Work out the finished part from the listing and answer in its coordinate system (mm). Round coordinates to 2 decimals unless told otherwise and drop trailing zeros. Loops run counter-clockwise (first coordinate to the right, second up) from the corner with the lowest first, then second, coordinate; pieces in that order, holes last. Notation, with made-up numbers: (-35, 45.25) - (-3, 45.25) arc R15 ccw to (-3, 59.25) - close; hole circle Ø3 at (5, 34). An arc over 180 degrees is marked (long way). Answer as CSV lines item,"result". Start each with the question number.
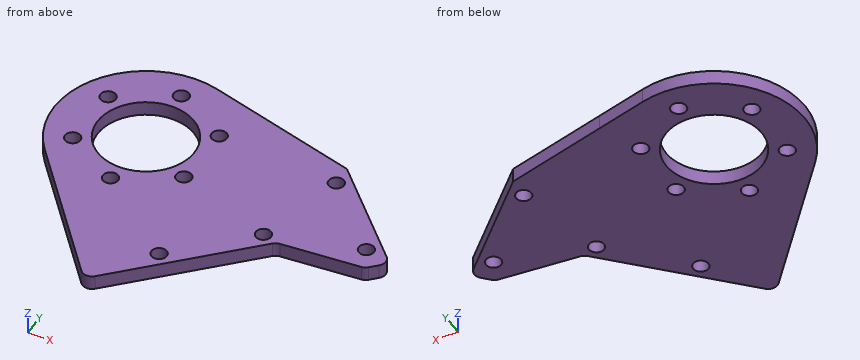
```python
from build123d import *

# Parameters (mm, degrees)
SKETCH_1_R          = 19
SKETCH_1_R_2        = 1.6
SKETCH_1_R_3        = 10
EXTRUDE_1_DEPTH     = 3
EXTRUDE_START       = -3
SKETCH_2_R          = 1.6
EXTRUDE_2_DEPTH     = 3
CUT_EXTRUDE_START   = -10
CUT_EXTRUDE_1_DEPTH = 10
EXTRUDE_4_DEPTH     = 3


with BuildPart() as part:
    # 草图1 → 凸台-拉伸1 (new body)
    with BuildSketch(Plane.XY):
        Circle(SKETCH_1_R)
        with Locations((0, 13.5)):
            Circle(SKETCH_1_R_2, mode=Mode.SUBTRACT)
        Circle(SKETCH_1_R_3, mode=Mode.SUBTRACT)
        with Locations((11.691342951, 6.75)):
            Circle(SKETCH_1_R_2, mode=Mode.SUBTRACT)
        with Locations((11.691342951, -6.75)):
            Circle(SKETCH_1_R_2, mode=Mode.SUBTRACT)
        with Locations((0, -13.5)):
            Circle(SKETCH_1_R_2, mode=Mode.SUBTRACT)
        with Locations((-11.691342951, -6.75)):
            Circle(SKETCH_1_R_2, mode=Mode.SUBTRACT)
        with Locations((-11.691342951, 6.75)):
            Circle(SKETCH_1_R_2, mode=Mode.SUBTRACT)
    extrude(amount=EXTRUDE_1_DEPTH)

    # 草图2 → 凸台-拉伸2 (add)
    with BuildSketch(Plane.XY.offset(3).offset(EXTRUDE_START)):
        with BuildLine():
            Line((24.748737342, 21.920310217), (55.507882323, -8.838834765))
            ThreePointArc((55.507882323, -8.838834765), (56.093668761, -10.253048327), (55.507882323, -11.66726189))
            Line((55.507882323, -11.66726189), (54.093668761, -13.081475452))
            ThreePointArc((54.093668761, -13.081475452), (53.524691722, -13.479877464), (52.853766684, -13.659651286))
            Line((52.853766684, -13.659651286), (36.481363532, -15.092050956))
            ThreePointArc((36.481363532, -15.092050956), (35.810438494, -15.271824778), (35.241461455, -15.67022679))
            Line((35.241461455, -15.67022679), (11.212279145, -39.699409101))
            ThreePointArc((11.212279145, -39.699409101), (9.707926642, -40.283163249), (8.262251105, -39.566317661))
            Line((8.262251105, -39.566317661), (-14.59023753, -12.170660163))
            ThreePointArc((-14.59023753, -12.170660163), (12.81586728, -14.026886535), (13.435028843, 13.435028843))
            Line((13.435028843, 13.435028843), (21.920310217, 21.920310217))
            ThreePointArc((21.920310217, 21.920310217), (23.334523779, 22.506096654), (24.748737342, 21.920310217))
        make_face()
        with Locations((51.265241636, -8.838834765)):
            Circle(SKETCH_2_R, mode=Mode.SUBTRACT)
        with Locations((37.123106012, 5.303300859)):
            Circle(SKETCH_2_R, mode=Mode.SUBTRACT)
        with Locations((18.384776311, -28.284271247)):
            Circle(SKETCH_2_R, mode=Mode.SUBTRACT)
        with Locations((32.526911935, -14.142135624)):
            Circle(SKETCH_2_R, mode=Mode.SUBTRACT)
    extrude(amount=EXTRUDE_2_DEPTH)

    # 草图5 → 切除-拉伸1 (cut)
    with BuildSketch(Plane.XY.offset(3).offset(CUT_EXTRUDE_START)):
        with BuildLine():
            Line((21.920310217, 21.920310217), (15.513435038, 15.513435038))
            Line((15.513435038, 15.513435038), (36.88104685, 9.788000708))
            Line((36.88104685, 9.788000708), (24.748737342, 21.920310217))
            ThreePointArc((24.748737342, 21.920310217), (23.334523779, 22.506096654), (21.920310217, 21.920310217))
        make_face()
    extrude(amount=CUT_EXTRUDE_1_DEPTH, mode=Mode.SUBTRACT)

    # 草图5<4> → 凸台-拉伸4 (add)
    with BuildSketch(Plane.XY.offset(3).offset(EXTRUDE_START)):
        with BuildLine():
            Line((15.513435038, 15.513435038), (4.917561857, 18.352590699))
            ThreePointArc((4.917561857, 18.352590699), (9.5, 16.454482672), (13.435028843, 13.435028843))
            Line((13.435028843, 13.435028843), (15.513435038, 15.513435038))
        make_face()
    extrude(amount=EXTRUDE_4_DEPTH)


solid = part.part
```
Item 1: Section D-D, the plane y = -34 is taken. Give the vertices of the cut face in (x, z).
Item 2: Find the intervals of material crossed by L1, parallel to X at y = 4, z = 0.9; L2, parallel to Y at x = 2, z = 1.7; L3, parallel to Y at x = -13, z = 0.4, in increasing order.
Item 3: Section A-A, the plane y = 13.5 is taken. Give the vertices of the cut face in (x, z).
Item 4: Section C-C, the plane z = 1.15 is taken. Count the separate pieces of the cut face and the enclosed holes in it, and give its area (3 significant figures).
Item 5: Section B-B, the plane x = 7 is taken. Give the vertices of the cut face in (y, z), and give its area (3 significant figures).
Answer:
1,outline,"(3.62, 0) - (16.91, 0) - (16.91, 3) - (3.62, 3) - close"
2,L1,"x = -18.57 to -9.17, 9.17 to 36.19, 38.05 to 42.67"
2,L2,"y = -32.06 to -9.8, 9.8 to 18.89"
2,L3,"y = -14.08 to -7.67, -5.83 to 5.83, 7.67 to 13.86"
3,outline,"(-13.37, 0) - (-1.6, 0) - (-1.6, 3) - (-13.37, 3) - close; (1.6, 0) - (23.03, 0) - (23.03, 3) - (1.6, 3) - close"
4,separate pieces,"1"
4,enclosed holes,"11"
4,area,"2,140 mm²"
5,outline,"(-38.05, 0) - (-7.14, 0) - (-7.14, 3) - (-38.05, 3) - close; (7.14, 0) - (17.79, 0) - (17.79, 3) - (7.14, 3) - close"
5,area,"125 mm²"
